Can you work these out from the model? Positions are in its coordinate system, mm. Face numbers are marked on the shaded views. A direction names the side the tool comes from. Coordinates: 2 decimals unless noted, no trailing zeros. Write each loop counter-clockwise with the first axis right and the second up, starting at its lowest first coordinate (ties: lowest second). Pieces come first, ordered by that corner, then holes. Notation, with made-up numbers: M 87,87.5 L 109,87.5 A13 cw 109,94.5 Z; hole C 19,80 d9. An arc over 180 degrees is marked long. Use one line per item in the form item = value. Start each with the question number.
Autodesk Inventor part; units mm, degrees
ref_plane "YZ Plane" through (0, 0, 0) normal (1, 0, 0) x (0, 1, 0)
ref_plane "XZ Plane" through (0, 0, 0) normal (0, 1, 0) x (-1, 0, 0)
ref_plane "XY Plane" through (0, 0, 0) normal (0, 0, 1) x (1, 0, 0)
sketch "Sketch1" plane through (0, 0, 0) normal (0, 0, 1) x (1, 0, 0)
  line L0 (2.1581, 5.715) -> (1.27, 5.715)
  line L1 (1.27, 5.715) -> (1.27, 0)
  line L2 (1.27, 0) -> (0, 0)
  line L3 (0, 0) -> (0, 7.62)
  arc A0 (2.3846, 6.084) -> (0, 7.62) centre (-0.1226, 4.8107) ccw
  arc A1 (2.1581, 5.715) -> (2.3846, 6.084) centre (2.1581, 5.969) ccw
  point P0 (2.54, 5.715)
  dimension "d0" = 7.62
  dimension "d1" = 2.54
  dimension "d2" = 1.905
  dimension "d3" = 1.27
  dimension "d4" = 0.254
revolve "Revolution1" add sketch "Sketch1" angle 360 about axis through (0, 0, 0) along (0, 1, 0)
sketch "Sketch2" plane through (0, 0, 0) normal (0, -1, 0) x (1, 0, 0)
  circle A0 centre (0, 0) radius 1.27
  line L0 (0.9525, 0.508) -> (0.508, 0.508)
  line L1 (0.508, 0.508) -> (0.508, 0.9525)
  line L2 (-0.508, 0.9525) -> (-0.508, 0.508)
  line L3 (-0.508, 0.508) -> (-0.9525, 0.508)
  line L4 (-0.9525, -0.508) -> (-0.508, -0.508)
  line L5 (-0.508, -0.508) -> (-0.508, -0.9525)
  line L6 (0.508, -0.9525) -> (0.508, -0.508)
  line L7 (0.9525, -0.508) -> (0.508, -0.508)
  arc A1 (0.9525, -0.508) -> (0.9525, 0.508) centre (0, 0) ccw
  arc A2 (-0.508, -0.9525) -> (0.508, -0.9525) centre (0, 0) ccw
  arc A3 (0.508, 0.9525) -> (-0.508, 0.9525) centre (0, 0) ccw
  arc A4 (-0.9525, 0.508) -> (-0.9525, -0.508) centre (0, 0) ccw
  point P0 (1.164, -0.508)
  point P1 (1.164, 0.508)
  point P2 (-1.164, -0.508)
  point P3 (-1.164, 0.508)
  point P4 (0.508, -1.164)
  point P5 (-0.508, -1.164)
  point P6 (-0.508, 1.164)
  point P7 (0.508, 1.164)
  dimension "d6" = 0.508
  dimension "d7" = 0.508
extrude "Extrusion1" cut sketch "Sketch2" against normal blind 25.4 contours A1 L7 L6 A2 L5 L4 A4 L3 L2 A3 L1 L0
sketch "Sketch3" plane through (0, 0, 0) normal (0, -1, 0) x (1, 0, 0)
  circle A0 centre (0, 0) radius 1.27
extrude "Extrusion2" add sketch "Sketch3" against normal blind 6.35
sketch "Sketch4" plane through (0, 0, 0) normal (0, -1, 0) x (1, 0, 0)
  circle A0 centre (0, 0) radius 1.27
extrude "Extrusion3" add sketch "Sketch4" along normal blind 4.445
properties part number "Screw"
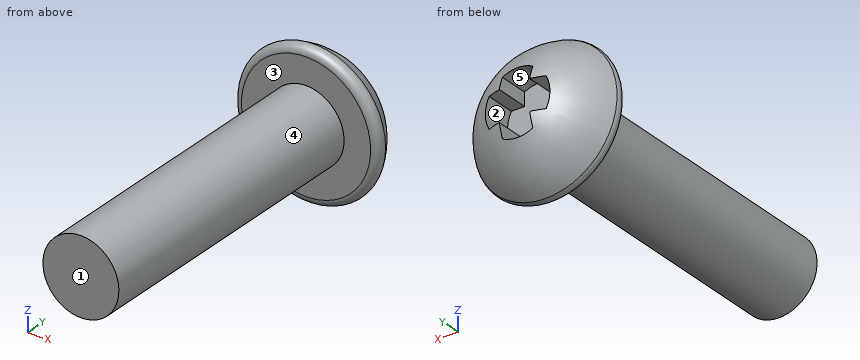
1) Suppose I cut it at A-A on y = 0. Please give me the cut outline in (x, z), and give its area (3 significant figures).
2) If we mould it in two halves opening along X, with no side actions, what happens to the marked faces 3, 4 and 5? For each: +X half, -X half, draft (parallel to the pull), parting line (faces both ways), or undercut.
3) Will these pins go through, and if not, where does the flat tip stop? pin 1 Ø0.5 at (x, y) = (0.5, 7) entering from -Z; pin 2 Ø1.1 at (x, z) = (0, 0) entering from +Y; pin 3 Ø1 at (y, z) = (-3, 0) entering from -X.
4) Which directions (+Z, -Z, +X, -X, +Y, -Y) give clear straight access to the entire face, cutting with the end or side of a thin tool? Please do the marked faces 1 and 2.
5) Please list where these lines run through material, in increasing order: line 1 (X direction, y = 4, z = -0.05); line 2 (Z direction, x = 1.15, y = 1); line 3 (Y direction, x = 0.65, z = -1.45) (3 decimals).
Computed values:
q1.outline = C 0,0 d2.54
q1.area = 5.07 mm²
q2.face_3 = draft
q2.face_4 = parting line
q2.face_5 = undercut
q3.pin_1 = -1.86
q3.pin_2 = 6.35
q3.pin_3 = -1.27
q4.face_1 = +Z, -Z, +X, -X, -Y
q4.face_2 = +Y
q5.line_1 = -1.27 to 1.27
q5.line_2 = -0.54 to 0.54
q5.line_3 = 5.715 to 7.042
